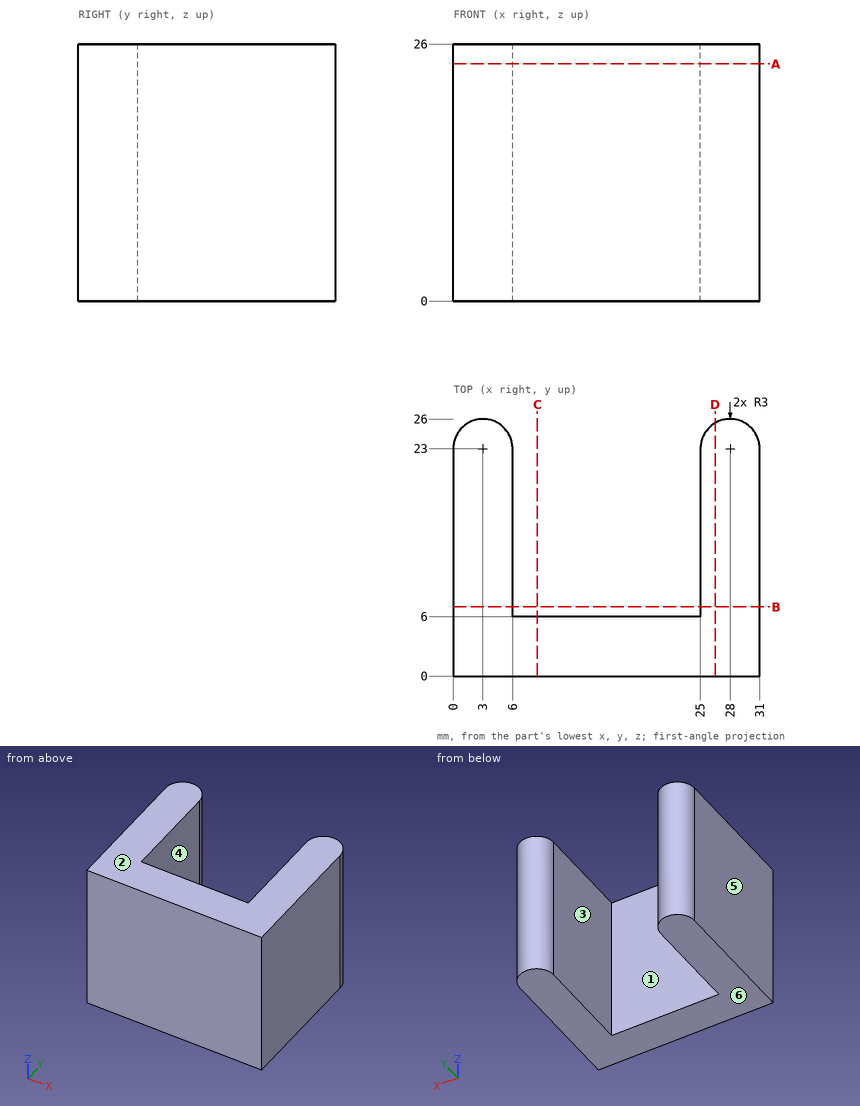
For this review, use the dimensioned drawing (mm, ordinates from the lowest corner) and the shaded views. A direction names the side the tool comes from. Round coordinates to 2 decimals unless told otherwise and drop trailing zeros. Loops run counter-clockwise (first coordinate to the right, second up) from the corner with the lowest first, then second, coordinate; pieces in that order, holes last. Notation, with made-up numbers: M 13.5,41 L 22.5,41 A30 ccw 22.5,66 Z; hole C 1,55 d10. An arc over 180 degrees is marked long. Answer as a JSON object with one key per item and string values.
(1) Take a section at A-A on z = 24. Give the boundary of the cut face in (x, y).
Resolved:
{"outline": "M 0,0 L 31,0 L 31,23 A3 ccw 25,23 L 25,6 L 6,6 L 6,23 A3 ccw 0,23 Z"}
(2) Take a section at C-C on x = 8.5. Give the boundary of the cut face in (y, z).
Resolved:
{"outline": "M 0,0 L 6,0 L 6,26 L 0,26 Z"}
(3) Tool access review of the marked faces 1 and 2: name each direction out of +Z, -Z, +X, -X, +Y, -Y from which nothing blocks a thin tool from reaching the whole face with its end or side.
Resolved:
{"face 1": "+Z, -Z, +Y", "face 2": "+Z, +X, -X, +Y, -Y"}
(4) Clearance check with a flat-ended pin moving along its axis: P1, Ø15, axis at x = 14, z = 11, coming from the +Y side. State where the tip first meets the part, or that it passes through.
Resolved:
{"P1": "y = 6"}
(5) Take a section at B-B on y = 7. Give the boundary of the cut face in (x, z).
Resolved:
{"outline": "M 0,0 L 6,0 L 6,26 L 0,26 Z; M 25,0 L 31,0 L 31,26 L 25,26 Z"}
(6) To check wall thickness, follow line 1 along X through (y, z) = (9, 14.5); line 2 along Y through (x, z) = (11.5, 13.5); line 3 along X through (y, z) = (24.5, 21.75). State the ranges of each line that lie inside material, in increasing order.
Resolved:
{"line 1": "0 to 6, 25 to 31", "line 2": "0 to 6", "line 3": "0.4 to 5.6, 25.4 to 30.6"}
(7) Take a section at D-D on x = 26.5. Give the boundary of the cut face in (y, z), and give its area (3 significant figures).
Resolved:
{"outline": "M 0,0 L 25.6,0 L 25.6,26 L 0,26 Z", "area": "666 mm²"}
(8) Draft analysis for pull direction X (two halves, no side actions). For the marked faces 3, 4, 5 and 6, state which applies: released by +X, released by -X, zero draft, split by the parting line, or undercut.
Resolved:
{"face 3": "undercut", "face 4": "undercut", "face 5": "released by -X", "face 6": "zero draft"}
